Check sheet for the modelled part. Datum: model origin and axes. Units: mm. A direction names the side the tool comes from. Round coordinates to 2 decimals unless told otherwise and drop trailing zeros. Order: outer loops, then holes, each group sorted by start corner. A loop starts at its lowest first (then second) coordinate and runs counter-clockwise, first axis right, second up. Notation, with made-up numbers: (44.5, 39) -> (79.5, 39) arc R31 ccw to (79.5, 77) -> close; hole circle Ø3 at (-19.5, 45). An arc over 180 degrees is marked (long way). Use CSV: the item, a comma, the result in double quotes.
```python
from build123d import *

# Parameters (mm, degrees)
BOSS_EXTRUDE2_DEPTH = 7.5
SKETCH3_W           = 19
SKETCH3_H           = 6
SKETCH3_R           = 1.75
BOSS_EXTRUDE3_DEPTH = 2
FILLET1_R           = 3


with BuildPart() as part:
    # Sketch2 → Boss-Extrude2 (new body)
    with BuildSketch(Plane.XY):
        Polygon((0, 9.5), (0, 0), (11.5, 0), (11.5, 9.5), (7.5, 9.5), (7.5, 3.5), (4, 3.5), (4, 9.5), align=None)
    extrude(amount=BOSS_EXTRUDE2_DEPTH)

    # Sketch3 → Boss-Extrude3 (add)
    with BuildSketch(Plane.ZY):
        with Locations((3.75, 3)):
            Rectangle(SKETCH3_W, SKETCH3_H)
        with Locations((-2.5, 3)):
            Circle(SKETCH3_R, mode=Mode.SUBTRACT)
        with Locations((10, 3)):
            Circle(SKETCH3_R, mode=Mode.SUBTRACT)
    extrude(amount=-BOSS_EXTRUDE3_DEPTH)

    # Fillet1
    fillet1_edges = [part.edges().sort_by_distance(p)[0] for p in [
        (1, 0, 13.25),
        (1, 6, 13.25),
        (1, 0, -5.75),
        (1, 6, -5.75),
    ]]
    fillet(fillet1_edges, radius=FILLET1_R - 0.0001)  # a hair under: the kernel refuses the full size


solid = part.part
```
Q1. Mould release check, pull along X, two halves, no side actions. Record for faces 6 (the face through (4, 6, 4)), 7 (the face through (8, 5, 0)), 8 (the face through (2, 1.7, -4.2)): pulls with the +X half, pulls with the -X half, needs draft (parallel to the pull), parting line crosses it, or undercut.
Result sheet:
face 6,"undercut"
face 7,"needs draft"
face 8,"pulls with the +X half"
Q2. Sectioned sample at B-B, the plane y = 7. Enter the section's corners in (x, z), then the cut area to 3 significant figures.
Result sheet:
outline,"(0, 0) -> (4, 0) -> (4, 7.5) -> (0, 7.5) -> close; (7.5, 0) -> (11.5, 0) -> (11.5, 7.5) -> (7.5, 7.5) -> close"
area,"60.0 mm^2"
Q3. Sectioned sample at D-D, the plane z = 4. Enter the section's corners in (x, y), then the cut area to 4 significant figures.
Result sheet:
outline,"(0, 0) -> (11.5, 0) -> (11.5, 9.5) -> (7.5, 9.5) -> (7.5, 3.5) -> (4, 3.5) -> (4, 9.5) -> (0, 9.5) -> close"
area,"88.25 mm^2"
Q4. Go/stop test with flat-tipped pins: pin 1 (2 mm diameter, centred on x = 2, y = 7.5, fed in from +Z); pin 2 (3 mm diameter, centred on x = 2, y = 6.5, fed in from +Z); pin 3 (4.5 mm diameter, centred on y = 3, z = -4.5, fed in from +X). Record where each tip stops, or that it passes through.
Result sheet:
pin 1,"stops at z = 7.5"
pin 2,"stops at z = 12.49"
pin 3,"stops at x = 2"
Q5. Access from +Z, -Z, +X, -X, +Y, -Y to the whole of each face (thin tool, end or side, straight path). Record for faces 1 (the face through (1.01, 0.9, -4.89)), 2 (the face through (1, 6, 9)), 3 (the face through (6, 3.5, 4)), 4 (the face through (1, 6, -1)), 5 (the face through (0, 4, 4)).
Result sheet:
face 1,"-Z, +X, -X, -Y"
face 2,"+Z, +X, -X, +Y"
face 3,"+Z, -Z, +Y"
face 4,"-Z, +X, -X, +Y"
face 5,"+Z, -Z, -X, +Y, -Y"
Q6. Scan lines: L1, parallel to Y at x = 0.7, z = 10; L2, parallel to X at y = 4.25, z = 0.5; L3, parallel to X at y = 0.5, z = 8.25. Record each from-to range of solid material in increasing order.
Result sheet:
L1,"y = 0 to 1.25, 4.75 to 6"
L2,"x = 0 to 4, 7.5 to 11.5"
L3,"x = 0 to 2"
Q7. Sectioned sample at C-C, the plane y = 2.5. Enter the section's corners in (x, z).
Result sheet:
outline,"(0, -5.71) -> (2, -5.71) -> (2, -4.18) -> (0, -4.18) -> close; (0, -0.82) -> (2, -0.82) -> (2, 0) -> (11.5, 0) -> (11.5, 7.5) -> (2, 7.5) -> (2, 8.32) -> (0, 8.32) -> close; (0, 11.68) -> (2, 11.68) -> (2, 13.21) -> (0, 13.21) -> close"
Q8. Sectioned sample at A-A, the plane z = 11. Enter the section's corners in (x, y), then the cut area to 3 significant figures.
Result sheet:
outline,"(0, 0.1) -> (2, 0.1) -> (2, 1.56) -> (0, 1.56) -> close; (0, 4.44) -> (2, 4.44) -> (2, 5.9) -> (0, 5.9) -> close"
area,"5.87 mm^2"
